from build123d import *

# Parameters (mm, degrees)
AUFSATZ_LINEAR_AUSTRAGEN1_DEPTH = 19
KREISMUSTER1_COUNT              = 5
KREISMUSTER1_ANGLE              = 60


with BuildPart() as part:
    # Skizze2 → Aufsatz-Linear austragen1 (new body)
    with BuildSketch(Plane.XY):
        Polygon((55.173482404, 0), (69.682060417, 14.508578013), (69.682060417, 0), align=None)
    aufsatz_linear_austragen1 = extrude(amount=-AUFSATZ_LINEAR_AUSTRAGEN1_DEPTH)

    # Kreismuster1: Aufsatz-Linear austragen1 ×5 about axis
    kreismuster1_axis = Axis((55.173482404, 0, 0), (0, -1, 0))
    for i in range(1, KREISMUSTER1_COUNT):
        add(aufsatz_linear_austragen1.rotate(kreismuster1_axis, i * KREISMUSTER1_ANGLE / (KREISMUSTER1_COUNT - 1)))


solid = part.part
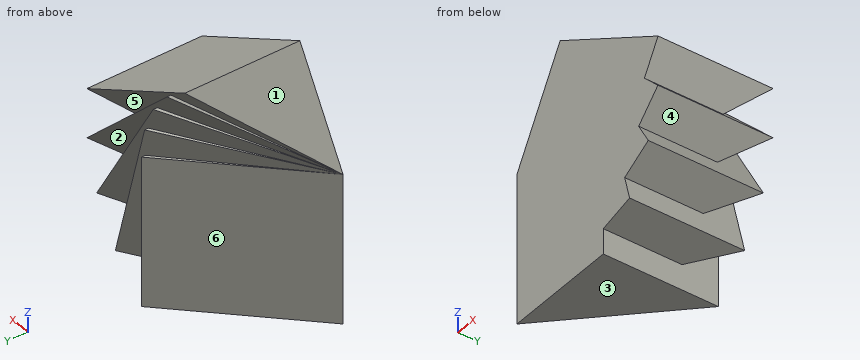
Verification items for the finished model (mm, model axes). Face numbers are marked on the shaded views. A direction names the side the tool comes from. Give positions to 0.01 mm unless a question says otherwise; leave off trailing zeros. Loops run counter-clockwise (first coordinate to the right, second up) from the corner with the lowest first, then second, coordinate; pieces in that order, holes last.
1) Depth check by flat-ended pin: pin 1 Ø12 at (x, z) = (68, -10) entering from +Y; pin 2 Ø4 at (y, z) = (5.5, -4) entering from +X; pin 3 Ø3 at (x, z) = (62, -14.5) entering from +Y. Enter the tip coordinate at first touch or a pass-through.
2) Draft check along X on the marked faces 1, 2 and 3. Enter one of: pulls with the +X half, pulls with the -X half, needs draft (parallel to the pull), parting line crosses it, or undercut.
3) Sectioned sample at C-C, the plane z = -8.5. Enter the section's corners in (x, y), then the cut area to 3 significant figures.
4) Sectioned sample at D-D, the plane y = 13.25. Enter the section's corners in (x, z) (1 decimal), then the cut area to 3 significant figures.
5) Thickness scan on line 1 along X through (y, z) = (7.25, -18); line 2 along Z through (x, y) = (77, 11); line 3 along X through (y, z) = (13.5, -14). Record the ranges inside material, lowest first.
6) Sectioned sample at B-B, the plane x = 66. Enter the section's corners in (y, z), then the cut area to 3 significant figures.
7) Set-up check for the marked faces 4, 5 and 6: record each of +Z, -Z, +X, -X, +Y, -Y from which the full face is reachable in a straight line by a thin tool's end or side.
Answers:
1. pin 1: stops at y = 14.51
1. pin 2: stops at x = 78.87
1. pin 3: stops at y = 8.33
2. face 1: pulls with the -X half
2. face 2: undercut
2. face 3: needs draft
3. outline: (55.17, 0) - (76.83, 0) - (76.83, 14.51) - (72.47, 10.73) - (72.47, 14.51) - (69.68, 11.81) - (69.68, 14.51) - close
3. area: 197 mm2
4. outline: (61.8, 11.5) - (64.9, 9.7) - (64.5, 9.4) - (67.1, 6.9) - (66.6, 6.6) - (68.4, 3.6) - (68, 3.4) - (68.9, 0) - (68.4, 0) - (68.4, -19) - (69.7, -19) - (69.7, -3) - (72.9, -14.9) - (74.1, -14.6) - (70, 0.9) - (76.1, -9.8) - (77.2, -9.2) - (69.2, 4.7) - (78, -4.1) - (78.9, -3.2) - (67.5, 8.2) - (78.3, 2) - (78.9, 3.1) - (62.4, 12.6) - close
4. area: 115 mm2
5. line 1: x = 62.42 to 69.68
5. line 2: z = -9.34 to -8.79, -5.04 to -1.31, 0.1 to 4.15
5. line 3: x = 68.67 to 69.68, 72.9 to 73.95
6. outline: (0, -19) - (10.83, -19) - (10.83, 0) - (10.46, 0) - (11.21, 2.9) - (10.83, 2.9) - (12.5, 6.25) - (12.08, 6.25) - (14.51, 9.69) - (13.81, 9.69) - (14.51, 10.5) - (0, 10.5) - close
6. area: 333 mm2
7. face 4: +X, +Y, -Y
7. face 5: +Y
7. face 6: -Z, -X, +Y
